```python
from build123d import *

# Parameters (mm, degrees)
SKETCH1_R                                       = 49.75
BOSS_EXTRUDE1_DEPTH                             = 3.175
CUT_EXTRUDE1_DEPTH                              = 71.428727271
SKETCH3_R                                       = 14
CUT_EXTRUDE2_DEPTH                              = 71.428727271
CIRPATTERN1_COUNT                               = 3
F_3_4_3_4_DIAMETER_HOLE1_D                      = 3.4
CIRPATTERN2_COUNT                               = 4
CSK_FOR_M3_FLAT_HEAD_MACHINE_SCREW2_D           = 3.4
CSK_FOR_M3_FLAT_HEAD_MACHINE_SCREW2_CSINK_D     = 6.3
CSK_FOR_M3_FLAT_HEAD_MACHINE_SCREW2_CSINK_ANGLE = 90
FILLET1_R                                       = 2
FILLET2_R                                       = 10
M3X0_5_TAPPED_HOLE1_D                           = 2.5


with BuildPart() as part:
    # Sketch1 → Boss-Extrude1 (new body)
    with BuildSketch(Plane(origin=(0, 0, 0), x_dir=(1, 0, 0), z_dir=(0, 1, 0))):
        with Locations(Location((0, 0, 0), (0, 0, 270))):
            Circle(SKETCH1_R)
    extrude(amount=BOSS_EXTRUDE1_DEPTH)

    # Sketch2 → Cut-Extrude1 (cut, through all)
    with BuildSketch(Plane(origin=(0, 3.175, 0), x_dir=(1, 0, 0), z_dir=(0, 1, 0))):
        with BuildLine():
            Line((14.25, 26.326806625), (14.25, -26.326806625))
            Line((14.25, -26.326806625), (39.136360913, -30.714943505))
            ThreePointArc((39.136360913, -30.714943505), (49.75, 0), (39.136360913, 30.714943505))
            Line((39.136360913, 30.714943505), (14.25, 26.326806625))
        make_face()
    extrude(amount=-CUT_EXTRUDE1_DEPTH, mode=Mode.SUBTRACT)

    # Sketch3 → Cut-Extrude2 (cut, through all)
    with BuildSketch(Plane(origin=(0, 3.175, 0), x_dir=(1, 0, 0), z_dir=(0, 1, 0))):
        with Locations(Location((-15.75, 0, 0), (0, 0, 270))):
            Circle(SKETCH3_R)
    extrude(amount=-CUT_EXTRUDE2_DEPTH, mode=Mode.SUBTRACT)

    # Sketch6 → CSK for M4 Flat Head Machine Screw1 (revolve, cut)
    with BuildSketch(Plane(origin=(5.75, 3.175, 0), x_dir=(0, 0, 1), z_dir=(1, 0, 0))):
        Polygon((0, 0), (0, 3.175), (2.25, 3.175), (2.25, 2.45), (4.7, 0), align=None)
    csk_for_m4_flat_head_machine_screw1 = revolve(axis=Axis((5.75, 9.525, 0), (0, -1, 0)), mode=Mode.SUBTRACT)

    # CirPattern1: CSK for M4 Flat Head Machine Screw1 ×3 about axis
    cirpattern1_axis = Axis((-15.75, 0, 0), (0, 1, 0))
    for i in range(1, CIRPATTERN1_COUNT):
        add(csk_for_m4_flat_head_machine_screw1.rotate(cirpattern1_axis, i * 360 / CIRPATTERN1_COUNT), mode=Mode.SUBTRACT)

    # 3.4 _3.4_ Diameter Hole1 (through all)
    with Locations(Plane(origin=(0, 0, 0), x_dir=(-1, 0, 0), z_dir=(0, -1, 0))):
        with Locations((-33.226947648, 33.226947648)):
            f_3_4_3_4_diameter_hole1 = Hole(F_3_4_3_4_DIAMETER_HOLE1_D / 2)

    # CirPattern2: 3.4 _3.4_ Diameter Hole1 ×4 about axis
    cirpattern2_axis = Axis((0, 0, 0), (0, 1, 0))
    for i in range(1, CIRPATTERN2_COUNT):
        add(f_3_4_3_4_diameter_hole1.rotate(cirpattern2_axis, i * 360 / CIRPATTERN2_COUNT), mode=Mode.SUBTRACT)

    # CSK for M3 Flat Head Machine Screw2 (through all)
    with Locations(Plane(origin=(0, 0, 0), x_dir=(-1, 0, 0), z_dir=(0, -1, 0))):
        with Locations((21.25, -34), (-10.75, -34), (-10.75, 34), (21.25, 34)):
            CounterSinkHole(CSK_FOR_M3_FLAT_HEAD_MACHINE_SCREW2_D / 2, CSK_FOR_M3_FLAT_HEAD_MACHINE_SCREW2_CSINK_D / 2, counter_sink_angle=CSK_FOR_M3_FLAT_HEAD_MACHINE_SCREW2_CSINK_ANGLE)

    # Fillet1
    fillet1_edges = [part.edges().sort_by_distance(p)[0] for p in [
        (39.136360913, 1.5875, -30.714943505),
        (39.136360913, 1.5875, 30.714943505),
    ]]
    fillet(fillet1_edges, radius=FILLET1_R)

    # Fillet2
    fillet2_edges = [part.edges().sort_by_distance(p)[0] for p in [
        (14.25, 1.5875, 26.326806625),
        (14.25, 1.5875, -26.326806625),
    ]]
    fillet(fillet2_edges, radius=FILLET2_R)

    # M3x0.5 Tapped Hole1 (through all)
    with Locations(Plane(origin=(0, 3.175, 0), x_dir=(1, 0, 0), z_dir=(0, 1, 0))):
        with Locations((-27.331300737, -37), (24.392621835, -39), (24.392621835, 39), (-27.331300737, 37)):
            Hole(M3X0_5_TAPPED_HOLE1_D / 2)


solid = part.part
```
Geometry: final body of the model. Coordinates: model frame, mm. A direction names the side the tool comes from. Round coordinates to 2 decimals unless told otherwise and drop trailing zeros. Order: outer loops, then holes, each group sorted by start corner. A loop starts at its lowest first (then second) coordinate and runs counter-clockwise, first axis right, second up. Notation, with made-up numbers: (4, -20) -> (23, -20) arc R20 ccw to (23, 5) -> close; hole circle Ø1 at (17.25, 55). An arc over 180 degrees is marked (long way). Use CSV: the item, a comma, the result in double quotes. Start each with the question number.
1) First-contact query: pin 1 Ø5.5 at (x, z) = (10.75, -34) entering from -Y; pin 2 Ø4 at (x, z) = (-21.25, -34) entering from +Y (3 decimals); pin 3 Ø5 at (x, z) = (5.75, 0) entering from +Y (3 decimals); pin 4 Ø1 at (y, z) = (2, -2.5) entering from -X. Flat tips, straight axial feed; report the tip coordinate or a pass-through.
2) Section A-A (z = 6). Return the cut outline in (x, y) (3 decimals), and give its area (3 significant figures).
3) Material intervals for line 1 along Z through (x, y) = (10.75, 2.4); line 2 along X through (y, z) = (2, 32.5); line 3 along Z through (x, y) = (-21.25, 2), sorted ascending. Write a range as from..to.
4) Section D-D (x = -44). Return the cut outline in (y, z) (3 decimals).
5) Draft query along X for faces 1 (the face through (-5.6, 0, 10.4)), 2 (the face through (11.53, 2.32, 35.51)), 3 (the face through (16.653, 1.565, -24.438)). Return one class per face: +X half, -X half, draft (parallel to the pull), parting line (faces both ways), or undercut.
6) Section C-C (x = 17). Return the cut outline in (y, z) (3 decimals), and give its area (3 significant figures).
7) Section B-B (y = 2.35). State how many separate pieces and enclosed holes the cut face has, and give its area (3 significant figures).
8) Set-up query: faces 4 (the face through (16.653, 1.565, 24.438)), 5 (the face through (-29.42, 1.61, -3.03)). Return all of +Z, -Z, +X, -X, +Y, -Y with unobstructed straight access to the full face (end or side cutting, diameter ignored); none if empty.
Returned:
1,pin 1,"stops at y = 0.4"
1,pin 2,"stops at y = 3.175"
1,pin 3,"stops at y = 0.975"
1,pin 4,"stops at x = -49.71"
2,outline,"(-49.387, 0) -> (-28.399, 0) -> (-28.399, 3.175) -> (-49.387, 3.175) -> close; (-3.101, 0) -> (14.25, 0) -> (14.25, 3.175) -> (-3.101, 3.175) -> close"
2,area,"122 mm²"
3,line 1,"z = -48.57..-35.7, -32.3..32.3, 35.7..48.57"
3,line 2,"x = -37.67..-34.76, -31.69..-22.05, -20.45..9.95, 11.55..31.69, 34.76..37.32"
3,line 3,"z = -44.98..-35.7, -32.3..-12.87, 12.87..32.3, 35.7..44.98"
4,outline,"(0, -23.218) -> (3.175, -23.218) -> (3.175, 23.218) -> (0, 23.218) -> close"
5,face 1,"draft"
5,face 2,"undercut"
5,face 3,"+X half"
6,outline,"(0, -46.755) -> (3.175, -46.755) -> (3.175, -24.823) -> (0, -24.823) -> close; (0, 24.823) -> (3.175, 24.823) -> (3.175, 46.755) -> (0, 46.755) -> close"
6,area,"139 mm²"
7,separate pieces,"1"
7,enclosed holes,"16"
7,area,"5,080 mm²"
8,face 4,"+X, +Y, -Y"
8,face 5,"+Y, -Y"
